The listing builds one solid part. Answer for the finished solid, in the listing's coordinates (mm). A direction names the side the tool comes from. Round coordinates to 2 decimals unless told otherwise and drop trailing zeros. Write each loop counter-clockwise with the first axis right and the second up, starting at its lowest first coordinate (ties: lowest second). Pieces come first, ordered by that corner, then holes.
from build123d import *

# Parameters (mm, degrees)
BOSS_EXTRUDE1_DEPTH = 10
SKETCH2_R           = 1.705
CUT_EXTRUDE1_DEPTH  = 15
SKETCH3_W           = 7.3
SKETCH3_H           = 8.65
CUT_EXTRUDE2_DEPTH  = 8
SKETCH4_R           = 1.705
CUT_EXTRUDE3_DEPTH  = 15
SKETCH5_W           = 7.3
SKETCH5_H           = 8.65
CUT_EXTRUDE4_DEPTH  = 8


with BuildPart() as part:
    # Sketch1 → Boss-Extrude1 (new body)
    with BuildSketch(Plane(origin=(0, 0, 0), x_dir=(1, 0, 0), z_dir=(0, 1, 0))):
        with BuildLine():
            Line((5, 50), (5, -50))
            Line((5, -50), (-30, -50))
            ThreePointArc((-30, -50), (-47.5, -32.5), (-30, -15))
            Line((-30, -15), (0, -15))
            Line((0, -15), (0, 15))
            Line((0, 15), (-30, 15))
            ThreePointArc((-30, 15), (-47.5, 32.5), (-30, 50))
            Line((-30, 50), (5, 50))
        make_face()
    extrude(amount=BOSS_EXTRUDE1_DEPTH)

    # Sketch2 → Cut-Extrude1 (cut)
    with BuildSketch(Plane.XY.offset(50)):
        with Locations((-6, 5)):
            Circle(SKETCH2_R)
    extrude(amount=-CUT_EXTRUDE1_DEPTH, mode=Mode.SUBTRACT)

    # Sketch3 → Cut-Extrude2 (cut)
    with BuildSketch(Plane.XY.offset(35)):
        with Locations((-6, 4.325)):
            Rectangle(SKETCH3_W, SKETCH3_H)
    extrude(amount=CUT_EXTRUDE2_DEPTH, mode=Mode.SUBTRACT)

    # Sketch4 → Cut-Extrude3 (cut)
    with BuildSketch(Plane(origin=(0, 0, -50), x_dir=(-1, 0, 0), z_dir=(0, 0, -1))):
        with Locations((6, 5)):
            Circle(SKETCH4_R)
    extrude(amount=-CUT_EXTRUDE3_DEPTH, mode=Mode.SUBTRACT)

    # Sketch5 → Cut-Extrude4 (cut)
    with BuildSketch(Plane(origin=(0, 0, -35), x_dir=(-1, 0, 0), z_dir=(0, 0, -1))):
        with Locations((6, 4.325)):
            Rectangle(SKETCH5_W, SKETCH5_H)
    extrude(amount=CUT_EXTRUDE4_DEPTH, mode=Mode.SUBTRACT)


solid = part.part
1. Section A-A on x = -21.5 is taken. Determine the outline of the cut face in (y, z), plus the area to 3 significant figures.
Geometry says:
outline: (0, -50) - (10, -50) - (10, -15) - (0, -15) - close; (0, 15) - (10, 15) - (10, 50) - (0, 50) - close
area: 700 mm2
2. A tool of negligible diameter and unlimited length cuts with its end or side. For faces 4 (the face through (-15, 5, -15)), 5 (the face through (-2.35, 4, -39)), 6 (the face through (-7.626, 5.512, -46.549)), 7 (the face through (-4.374, 5.512, 46.549)), from which of +Z, -Z, +X, -X, +Y, -Y can it reach the whole face along a straight path? Write none if from no direction.
Geometry says:
face 4: -X, +Y, -Y
face 5: -Y
face 6: -Z
face 7: +Z
3. Straight lines are drawn through the part: line 1 along Z through (x, y) = (-9.5, 1); line 2 along Y through (x, z) = (-6, 46) (3 decimals); line 3 along Z through (x, y) = (-5, 5.25). For each, find the intervals that lie inside material, in ascending order.
Geometry says:
line 1: z = -50 to -43, -35 to -15, 15 to 35, 43 to 50
line 2: y = 0 to 3.295, 6.705 to 10
line 3: z = -35 to -15, 15 to 35
4. For a pull along X with two mould halves and no side action, classify faces 1 (the face through (-15, 5, 15)), 2 (the face through (-6, 4, 35)), 3 (the face through (0, 5, 0)) as released by +X, released by -X, zero draft, split by the parting line, or undercut.
Geometry says:
face 1: zero draft
face 2: undercut
face 3: released by -X
5. Section C-C on y = 5 is taken. Determine the outline of the cut face in (x, z) (3 decimals), plus the area to 3 significant figures.
Geometry says:
outline: (-30, -50) - (-7.705, -50) - (-7.705, -43) - (-9.65, -43) - (-9.65, -35) - (-2.35, -35) - (-2.35, -43) - (-4.295, -43) - (-4.295, -50) - (5, -50) - (5, 50) - (-4.295, 50) - (-4.295, 43) - (-2.35, 43) - (-2.35, 35) - (-9.65, 35) - (-9.65, 43) - (-7.705, 43) - (-7.705, 50) - (-30, 50) arc R17.5 ccw to (-30, 15) - (0, 15) - (0, -15) - (-30, -15) arc R17.5 ccw to start
area: 3,400 mm2
6. Section B-B on x = -6 is taken. Determine the outline of the cut face in (y, z) (3 decimals).
Geometry says:
outline: (0, -50) - (3.295, -50) - (3.295, -43) - (0, -43) - close; (0, -35) - (8.65, -35) - (8.65, -43) - (6.705, -43) - (6.705, -50) - (10, -50) - (10, -15) - (0, -15) - close; (0, 15) - (10, 15) - (10, 50) - (6.705, 50) - (6.705, 43) - (8.65, 43) - (8.65, 35) - (0, 35) - close; (0, 43) - (3.295, 43) - (3.295, 50) - (0, 50) - close
7. Section D-D on x = -36 is taken. Determine the outline of the cut face in (y, z), plus the area to 3 significant figures.
Geometry says:
outline: (0, -48.94) - (10, -48.94) - (10, -16.06) - (0, -16.06) - close; (0, 16.06) - (10, 16.06) - (10, 48.94) - (0, 48.94) - close
area: 658 mm2
8. Given pin 1 (2.5 mm diameter, centred on x = -6, y = 5, fed in from -Z); pin 2 (2.5 mm diameter, centred on y = 6, z = 40.5, fed in from -X); pin 3 (4 mm diameter, centred on x = -37, y = 1.5, fed in from +Z), each flat-ended and moving along its own axis, determine where each tip first touches the part or whether it passes through.
Geometry says:
pin 1: stops at z = -35
pin 2: stops at x = -46.15
pin 3: stops at z = 49.27
